Build history of the part. All positions in model axes, mm. A direction names the side the tool comes from. Give positions to 0.01 mm unless a question says otherwise; leave off trailing zeros. Loops run counter-clockwise (first coordinate to the right, second up) from the corner with the lowest first, then second, coordinate; pieces in that order, holes last. Notation, with made-up numbers: (9.5, -10) -> (64.5, -10) arc R20 ccw to (64.5, 9) -> close; hole circle Ø4 at (-20, -24.75). An arc over 180 degrees is marked (long way). Answer as a JSON object with one key per item and string values. Group by question number.
Q1. Band-saw the part on D-D, the plane y = 64. Write the cut outline in (x, z).
Q2. Band-saw the part on C-C, the plane x = 16.5. Write the cut outline in (y, z), plus the area to 3 significant figures.
Q3. Two-plate mould, pull along X, no slides. Class faces 1 (the cylindrical face through (6.466, -8.406, 9.675)), 2 (the flat face through (0, 4.525, 13)), 3 (the cylindrical face through (-17.776, -85.775, -1.479)): pulls with the +X half, pulls with the -X half, needs draft (parallel to the pull), parting line crosses it, or undercut.
Q4. Band-saw the part on A-A, the plane x = 0. Write the cut outline in (y, z) (3 decimals).
Q5. Drop flat-ended pins along their axis: pin 1 (3 mm diameter, centred on x = 0, z = 14, fed in from +Y) (3 decimals); pin 2 (0.8 mm diameter, centred on y = 4, z = 8.5, fed in from -X); pin 3 (8 mm diameter, centred on x = 42.5, z = 0.5, fed in from -Y). Give the stop position or say it passes through.
Q6. Wall check: probe 1 along Y at (x, z) = (4.5, 11.75); probe 2 along Z at (x, y) = (-1.5, -74); probe 3 along X at (y, z) = (4, 3.5). Give the ranges that are in metal, low to high. Write a range as from..to.
Q7. Band-saw the part on B-B, the plane z = 11. Write the cut outline in (x, y) (3 decimals), plus the area to 3 significant figures.
Q8. Tool access for faces 4 (the flat face through (-19, 14, 0)), 5 (the flat face through (-4, 1, 22)): list every direction of +Z, -Z, +X, -X, +Y, -Y with a clear straight run to the whole face (end or side of a thin tool).
from build123d import *

# Parameters (mm, degrees)
F0_R      = 82
F1_DEPTH  = 3
F2_R      = 26.9
F3_DEPTH  = 3
F4_R      = 9.45
F5_DEPTH  = 19
F6_W      = 4
F6_H      = 11.45
F7_DEPTH  = 19
F9_DEPTH  = 20
F9_FACE_W = 4
F9_FACE_H = 19
F10_DEPTH = 1.2
F11_R     = 7
F12_DEPTH = 25


with BuildPart() as f1:
    # F0 (on Top) → F1 (new body)
    with BuildSketch(Plane.XY):
        Circle(F0_R)
    extrude(amount=-F1_DEPTH)

    # F2 (on face) → F3 (join)
    with BuildSketch(Plane.XY):
        Circle(F2_R)
    extrude(amount=F3_DEPTH)

    # F4 (on face) → F5 (join)
    with BuildSketch(Plane.XY.offset(3)):
        Circle(F4_R)
    extrude(amount=F5_DEPTH)

    # F6 (on face) → F7 (join)
    with BuildSketch(Plane.XY.offset(22)):
        Rectangle(F6_W, F6_H)
    extrude(amount=-F7_DEPTH)


with BuildPart() as f1_1:
    # F8: moved
    add(f1.part.moved(Location((0, -5.725, 0))))

    # F6 (on face) → F9 (join)
    with BuildSketch(Plane.XY.offset(22)):
        Rectangle(F6_W, F6_H)
    extrude(amount=-F9_DEPTH)

    # F9_face (on face) → F10 (cut)
    with BuildSketch(Plane(origin=(0, 5.725, 12.5), x_dir=(-1, 0, 0), z_dir=(0, 1, 0))):
        Rectangle(F9_FACE_W, F9_FACE_H)
    extrude(amount=-F10_DEPTH, mode=Mode.SUBTRACT)

    # F11 (on face) → F12 (cut)
    with BuildSketch(Plane.XY.offset(22)):
        with Locations((0, -5.725)):
            Circle(F11_R)
    extrude(amount=-F12_DEPTH, mode=Mode.SUBTRACT)


solid = f1_1.part
Worked answers:
{
 "1": {"outline": "(-43.16, -3) -> (43.16, -3) -> (43.16, 0) -> (-43.16, 0) -> close"},
 "2": {"outline": "(-86.05, -3) -> (74.6, -3) -> (74.6, 0) -> (15.52, 0) -> (15.52, 3) -> (-26.97, 3) -> (-26.97, 0) -> (-86.05, 0) -> close", "area": "609 mm2"},
 "3": {"face 1": "undercut", "face 2": "needs draft", "face 3": "parting line crosses it"},
 "4": {"outline": "(-87.725, -3) -> (-12.725, -3) -> (-12.725, 22) -> (-15.175, 22) -> (-15.175, 3) -> (-32.625, 3) -> (-32.625, 0) -> (-87.725, 0) -> close; (1.275, -3) -> (76.275, -3) -> (76.275, 0) -> (21.175, 0) -> (21.175, 3) -> (4.525, 3) -> (4.525, 22) -> (1.275, 22) -> close"},
 "5": {"pin 1": "y = 4.525", "pin 2": "x = -2", "pin 3": "y = -78.11"},
 "6": {"probe 1": "-14.03..-11.09, -0.36..2.58", "probe 2": "-3..0", "probe 3": "-2..2"},
 "7": {"outline": "(-2, 3.511) arc R9.45 ccw (long way) to (2, 3.511) -> (2, 4.525) -> (-2, 4.525) -> close; hole circle Ø14 at (0, -5.725)", "area": "130 mm2"},
 "8": {"face 4": "+Z", "face 5": "+Z, +X, -X, +Y, -Y"}
}
